Design review of the part built by this model. Coordinates are the model's own, in mm. Coordinates: 2 decimals unless noted, no trailing zeros. Write each loop counter-clockwise with the first axis right and the second up, starting at its lowest first coordinate (ties: lowest second). Pieces come first, ordered by that corner, then holes. Notation, with made-up numbers: M 52,-32 L 65,-32 A21 cw 65,-18 Z; hole C 52.5,73 d1. An arc over 180 degrees is marked long. One line per question, with ' | ' between items.
from build123d import *

# Parameters (mm, degrees)
BOSS_EXTRUDE1_DEPTH = 904
SKETCH4_W           = 904
SKETCH4_H           = 26.674416974
CUT_EXTRUDE3_DEPTH  = 10
SKETCH7_R           = 5
BOSS_EXTRUDE4_DEPTH = 5


with BuildPart() as part:
    # Sketch1 → Boss-Extrude1 (new body)
    with BuildSketch(Plane.XY):
        Polygon((0, 35), (5, 35), (5, 30), (10, 30), (10, 35), (15, 35), (15, 0), (0, 0), align=None)
    extrude(amount=BOSS_EXTRUDE1_DEPTH)

    # Sketch4 → Cut-Extrude3 (cut)
    with BuildSketch(Plane.ZY):
        with Locations((452, 13.337208487)):
            Rectangle(SKETCH4_W, SKETCH4_H)
    extrude(amount=-CUT_EXTRUDE3_DEPTH, mode=Mode.SUBTRACT)

    # Sketch7 → Boss-Extrude4 (add)
    with BuildSketch(Plane.ZY.offset(-10)):
        with Locations((304, 12.5)):
            Circle(SKETCH7_R)
    extrude(amount=BOSS_EXTRUDE4_DEPTH)


solid = part.part
1. Insertion check: pin 1 Ø11 at (y, z) = (10.5, 302) entering from -X; pin 2 Ø3 at (x, z) = (6, 567) entering from -Y; pin 3 Ø2.5 at (y, z) = (31.5, 348) entering from -X; pin 4 Ø8 at (y, z) = (7.5, 109.5) entering from -X. Each pin has a flat end and moves straight along its axis. Give the tip position at first contact, or say it passes through.
Answer sheet:
pin 1: x = 5 | pin 2: y = 26.67 | pin 3: x = 0 | pin 4: x = 10
2. To check wall thickness, follow line 1 along X through (y, z) = (31.5, 115.5); line 2 along Y through (x, z) = (6, 194); line 3 along X through (y, z) = (25, 396.5). State the ranges of each line that lie inside material, in increasing order. Write a range as [from, to].
Answer sheet:
line 1: [0, 5], [10, 15] | line 2: [26.67, 30] | line 3: [10, 15]
3. Take a section at A-A (z = 448.5). Write out the cut boundary in (x, y), then the cut area to 3 significant figures.
Answer sheet:
outline: M 0,26.67 L 10,26.67 L 10,0 L 15,0 L 15,35 L 10,35 L 10,30 L 5,30 L 5,35 L 0,35 Z | area: 233 mm^2
